from build123d import *

# Parameters (mm, degrees)
F0_R     = 15.875
F1_DEPTH = 152.4
F3_D     = 12
F3_DEPTH = 32
F3_TIP   = 3.6051637142
F4_W     = 18
F4_H     = 4
F5_DEPTH = 8.5
F6_R     = 15.875
F6_R_2   = 9.525
F7_DEPTH = 127


with BuildPart() as f1:
    # F0 (on Right) → F1 (new body)
    with BuildSketch(Plane.YZ):
        Circle(F0_R)
    extrude(amount=F1_DEPTH)

    # F3
    with Locations(Plane(origin=(0, 0, 0), x_dir=(0, -1, 0), z_dir=(-1, 0, 0))):
        with Locations((0, 0)):
            Hole(F3_D / 2, depth=F3_DEPTH)
            with Locations((0, 0, -(F3_DEPTH + F3_TIP / 2))):  # 118° drill point
                Cone(0, F3_D / 2, F3_TIP, mode=Mode.SUBTRACT)

    # F4 (on Top) → F5 (cut)
    with BuildSketch(Plane.XY):
        with Locations((9, 0)):
            Rectangle(F4_W, F4_H)
    extrude(amount=F5_DEPTH, mode=Mode.SUBTRACT)

    # F6 (on face) → F7 (cut)
    with BuildSketch(Plane.YZ.offset(152.4)):
        Circle(F6_R)
        Circle(F6_R_2, mode=Mode.SUBTRACT)
    extrude(amount=-F7_DEPTH, mode=Mode.SUBTRACT)


solid = f1.part
Model file for the job. Use its own axes, mm. A direction names the side the tool comes from. Round coordinates to 2 decimals unless told otherwise and drop trailing zeros. Loops run counter-clockwise (first coordinate to the right, second up) from the corner with the lowest first, then second, coordinate; pieces in that order, holes last.
1. Wall check: probe 1 along Z at (x, y) = (25, 0) (3 decimals); probe 2 along Z at (x, y) = (14, 0) (3 decimals); probe 3 along Z at (x, y) = (49, 0.5). Give the ranges that are in metal, low to high.
Check values:
probe 1: z = -15.875 to -6, 6 to 15.875
probe 2: z = -15.875 to -6, 8.5 to 15.875
probe 3: z = -9.51 to 9.51
2. Tool access for faces 1 (the flat face through (18, 0, 7)), 2 (the flat face through (152.4, 0, 0)), 3 (the cylindrical face through (89.789, -7.559, -5.796)): list every direction of +Z, -Z, +X, -X, +Y, -Y with a clear straight run to the whole face (end or side of a thin tool).
Check values:
face 1: -X
face 2: +Z, -Z, +X, +Y, -Y
face 3: +X
3. Mould opens along Z. For faces 4 (the flat face through (9, -2, 7)), 5 (the cylindrical face through (12.522, -3.441, -15.497)), 6 (the flat face through (25.4, 7, -7)), 7 (the conical face through (34.98, -0.96, -0.4)) say: +Z half, -Z half, draft (parallel to the pull), parting line (faces both ways), or undercut.
Check values:
face 4: undercut
face 5: parting line
face 6: draft
face 7: undercut
4. Band-saw the part on D-D, the plane z = 11. List the corners of the cut face in (x, y), and give its area (3 significant figures).
Check values:
outline: (0, -11.45) - (25.4, -11.45) - (25.4, 11.45) - (0, 11.45) - close
area: 581 mm2
5. Band-saw the part on B-B, the plane y = 8. List the corners of the cut face in (x, z), and give its area (3 significant figures).
Check values:
outline: (0, -13.71) - (25.4, -13.71) - (25.4, -5.17) - (152.4, -5.17) - (152.4, 5.17) - (25.4, 5.17) - (25.4, 13.71) - (0, 13.71) - close
area: 2,010 mm2
6. Band-saw the part on A-A, the plane x = 14. List the corners of the cut face in (y, z) (3 decimals).
Check values:
outline: circle Ø31.75 at (0, 0); hole (-2, 5.657) arc R6 ccw (long way) to (2, 5.657) - (2, 8.5) - (-2, 8.5) - close
7. Band-saw the part on C-C, the plane x = 42. List the corners of the cut face in (y, z) (3 decimals), and give its area (3 significant figures).
Check values:
outline: circle Ø19.05 at (0, 0)
area: 285 mm2
8. Drop flat-ended pins along their axis: P1, Ø3, axis at x = 117.5, y = -9.5, coming from the -Z side; P2, Ø3, axis at x = 86, z = -3, coming from the -Y side; P3, Ø2, axis at x = 80.5, z = 4.5, coming from the +Y side. Give the stop position or say it passes through.
Check values:
P1: stops at z = -5.17
P2: stops at y = -9.41
P3: stops at y = 8.86
